Build history of the part. All positions in model axes, mm. Coordinates: 2 decimals unless noted, no trailing zeros. Write each loop counter-clockwise with the first axis right and the second up, starting at its lowest first coordinate (ties: lowest second). Pieces come first, ordered by that corner, then holes. Notation, with made-up numbers: (17, 25) -> (47, 25) arc R4 cw to (47, 30) -> close; hole circle Ø2 at (4, 39.25). An arc over 180 degrees is marked (long way). Write each question's results on one line, items separated by ' | '. Start each with the question number.
Q1. Saw through at C-C on x = -16. Give the cut face in (y, z).
Q2. Two-plate mould, pull along X, no slides. Class faces 1 (the face through (27.232, -23.162, 0.783)), 2 (the face through (21.735, -12.307, 0.783)), 3 (the face through (-1.09, -7.98, 0.78)): released by +X, released by -X, zero draft, split by the parting line, or undercut.
Q3. Saw through at D-D on y = -16. Give the cut face in (x, z).
Q4. Drill centre lines: line 1 (X direction, y = 13.5, z = 0.3); line 2 (Y direction, x = -20.5, z = 1.45); line 3 (Y direction, x = -20, z = 0.2). Where is each one in solid material? Low to high.
Q5. Saw through at A-A on y = -11. Count the separate pieces of the cut face and the enclosed holes in it, and give its area (3 significant figures).
Autodesk Inventor part; units mm, degrees
ref_plane "YZ Plane" through (0, 0, 0) normal (1, 0, 0) x (0, 1, 0)
ref_plane "XZ Plane" through (0, 0, 0) normal (0, 1, 0) x (-1, 0, 0)
ref_plane "XY Plane" through (0, 0, 0) normal (0, 0, 1) x (1, 0, 0)
sketch "Sketch1" plane through (0, 0, 0) normal (0, 0, 1) x (1, 0, 0)
  circle A0 centre (23.9168, 13.1886) radius 2.1844
  ellipse E0 centre (12.3891, -9.6575) end of major axis (10.2047, -9.6575) minor radius 2.1844
  ellipse E1 centre (-18.832, 12.1795) end of major axis (-21.0164, 12.1795) minor radius 2.1844
  line L0 (-18.832, 18.5295) -> (23.7667, 19.5368)
  arc A1 (-18.832, 18.5295) -> (-22.4715, 6.9759) centre (-18.832, 12.1795) ccw
  arc A2 (30.2668, 13.1886) -> (23.7667, 19.5368) centre (23.9168, 13.1886) ccw
  line L1 (-22.4715, 6.9759) -> (20.8933, -23.3546)
  line L2 (30.2668, 13.1886) -> (30.2458, -17.7636)
  arc A3 (20.8933, -23.3546) -> (30.2458, -17.7636) centre (23.8958, -17.7593) ccw
  circle A4 centre (23.9168, -12.2114) radius 2.1844
  point P0 (0, 0)
  dimension "d6" = 4.3688
extrude "Extrusion2" add sketch "Sketch1" along normal blind 1.5875
Returned:
1) outline: (2.45, 0) -> (18.6, 0) -> (18.6, 1.59) -> (2.45, 1.59) -> close
2) face 1: split by the parting line | face 2: undercut | face 3: released by -X
3) outline: (10.38, 0) -> (30.25, 0) -> (30.25, 1.59) -> (10.38, 1.59) -> close
4) line 1: x = -25.04 to -20.57, -17.09 to 21.75, 26.08 to 30.26 | line 2: y = 5.6 to 10.77, 13.59 to 18.31 | line 3: y = 5.25 to 10.33, 14.03 to 18.42
5) separate pieces: 3 | enclosed holes: 0 | area: 31.7 mm2
